Can you work these out from the model? Positions are in its coordinate system, mm. A direction names the side the tool comes from. Round coordinates to 2 decimals unless told otherwise and drop trailing zeros. Write each loop counter-clockwise with the first axis right and the second up, starting at its lowest first coordinate (ties: lowest second). Pieces come first, ordered by that corner, then holes.
Q1. We'd pull the mould along Y, two halves only. Please class faces 5 (the cylindrical face through (3.545, -3.18, 6.228)), 6 (the flat face through (0, 3.624, 3)), 7 (the flat face through (0, -3, 4.424)): +Y half, -Y half, draft (parallel to the pull), parting line (faces both ways), or undercut.
Q2. I'm going to push flat-ended pins straight in: pin 1 Ø0.8 at (x, y) = (0, -3) entering from +Z; pin 2 Ø1.1 at (x, z) = (-1, -0.5) entering from -Y; pin 3 Ø0.5 at (x, y) = (3, -3.5) entering from +Z; pin 4 Ø1.2 at (x, z) = (1, -1) entering from -Y. Where does each tip first touch, or does it pass through?
Q3. If we section it at A-A (z = 4.25): Please give me the cut outline in (x, y).
Q4. For faces 1 (the flat face through (0, -3.124, -1)), 2 (the cylindrical face through (-7.886, 0.069, -0.74)), 3 (the flat face through (0, 3.124, -1)), 4 (the cylindrical face through (6.926, -0.048, -0.291)), which set-ups out of +Z, -Z, +X, -X, +Y, -Y let a thin tool reach every point of the face, with its end or its side?
Q5. If we section it at B-B (y = 0): Please give me the cut outline in (x, z).
Q6. Please list where these lines run through material, in increasing order: line 1 along Y through (x, z) = (4.5, 3); line 2 along X through (y, z) = (0, 5.5); line 3 along Z through (x, y) = (-5.5, -1.25).
from build123d import *
from OCP.BRepAlgoAPI import BRepAlgoAPI_Cut
from OCP.TopTools import TopTools_ListOfShape

# Parameters (mm, degrees)
BOSS_EXTRUDE1_DEPTH      = 1.5
BOSS_EXTRUDE3_DEPTH      = 0.5
BOSS_EXTRUDE3_DRAFT      = -45
BOSS_EXTRUDE4_DEPTH      = 6.8
SHELL1_T                 = -0.96
SHELL1_THICKNESS_2_DEPTH = 0.46
CUT_EXTRUDE1_START       = -2.114122
CUT_EXTRUDE1_DEPTH       = 2.114122
SKETCH5_W                = 2.54
SKETCH5_H                = 7.2484
CUT_EXTRUDE2_DEPTH       = 0.762


with BuildPart() as part:
    # Sketch2 → Boss-Extrude1 (new body)
    with BuildSketch(Plane.XY):
        with BuildLine():
            Line((-4.7625, -3.1242), (4.7625, -3.1242))
            ThreePointArc((4.7625, -3.1242), (7.8867, 0), (4.7625, 3.1242))
            Line((4.7625, 3.1242), (-4.7625, 3.1242))
            ThreePointArc((-4.7625, 3.1242), (-7.8867, 0), (-4.7625, -3.1242))
        make_face()
    extrude(amount=-BOSS_EXTRUDE1_DEPTH)


with BuildPart() as boss_extrude3_tool:
    # Sketch2<3> → Boss-Extrude3 (with draft: the straight prism first)
    with BuildSketch(Plane.XY):
        with BuildLine():
            Line((-4.7625, -3.1242), (4.7625, -3.1242))
            ThreePointArc((4.7625, -3.1242), (7.8867, 0), (4.7625, 3.1242))
            Line((4.7625, 3.1242), (-4.7625, 3.1242))
            ThreePointArc((-4.7625, 3.1242), (-7.8867, 0), (-4.7625, -3.1242))
        make_face()
    extrude(amount=BOSS_EXTRUDE3_DEPTH)
    # Boss-Extrude3: the draft: its side faces are tilted about the plane it starts from
    boss_extrude3_sides = [boss_extrude3_tool.faces().sort_by_distance(p)[0] for p in [
        (0, -3.1242, 0.25),
        (7.8867, 0, 0.25),
        (0, 3.1242, 0.25),
        (-7.8867, 0, 0.25),
    ]]
    draft(boss_extrude3_sides, Plane.XY, BOSS_EXTRUDE3_DRAFT)


with BuildPart() as part_1:
    add(part.part)

    # Boss-Extrude3: add boss_extrude3_tool
    add(boss_extrude3_tool.part)

    # Sketch3 → Boss-Extrude4 (add)
    with BuildSketch(Plane.XY.offset(0.5)):
        with BuildLine():
            Line((-4.7625, -3.6242), (4.7625, -3.6242))
            ThreePointArc((4.7625, -3.6242), (8.3867, 0), (4.7625, 3.6242))
            Line((4.7625, 3.6242), (-4.7625, 3.6242))
            ThreePointArc((-4.7625, 3.6242), (-8.3867, 0), (-4.7625, -3.6242))
        make_face()
    extrude(amount=BOSS_EXTRUDE4_DEPTH)

    # Shell1
    shell1_openings = [part_1.faces().sort_by_distance(p)[0] for p in [
        (0, 0, 7.3),
    ]]
    offset(amount=SHELL1_T, openings=shell1_openings, kind=Kind.INTERSECTION)

    # Shell1 thickness 2 face (on inner face of the shell) → Shell1 thickness 2 (cut)
    with BuildSketch(Plane(origin=(0, 0, -0.54), x_dir=(-1, 0, 0), z_dir=(0, 0, -1))):
        with BuildLine():
            Line((-4.7625, 2.1642), (4.7625, 2.1642))
            ThreePointArc((4.7625, 2.1642), (6.9267, 0), (4.7625, -2.1642))
            Line((4.7625, -2.1642), (-4.7625, -2.1642))
            ThreePointArc((-4.7625, -2.1642), (-6.9267, 0), (-4.7625, 2.1642))
        make_face()
    extrude(amount=SHELL1_THICKNESS_2_DEPTH, mode=Mode.SUBTRACT)

    # Sketch4 → Cut-Extrude1 (cut)
    with BuildSketch(Plane.XY.offset(7.3).offset(CUT_EXTRUDE1_START)):
        with BuildLine():
            Line((1.3335, 4.572), (-1.3335, 4.572))
            ThreePointArc((-1.3335, 4.572), (-3.367596045, 3.367596045), (-4.572, 1.3335))
            Line((-4.572, 1.3335), (-4.572, -1.3335))
            ThreePointArc((-4.572, -1.3335), (-3.367596045, -3.367596045), (-1.3335, -4.572))
            Line((-1.3335, -4.572), (1.3335, -4.572))
            ThreePointArc((1.3335, -4.572), (3.367596045, -3.367596045), (4.572, -1.3335))
            Line((4.572, -1.3335), (4.572, 1.3335))
            ThreePointArc((4.572, 1.3335), (3.367596045, 3.367596045), (1.3335, 4.572))
        make_face()
    extrude(amount=CUT_EXTRUDE1_DEPTH, mode=Mode.SUBTRACT)


with BuildPart() as cut_extrude2_tool:
    # Sketch5 → Cut-Extrude2 (new body)
    with BuildSketch(Plane.XY.offset(5.185877531)):
        Rectangle(SKETCH5_W, SKETCH5_H)
    extrude(amount=-CUT_EXTRUDE2_DEPTH)


with BuildPart() as part_2:
    add(part_1.part)

    # Cut-Extrude2: cut by cut_extrude2_tool, with a tolerance
    cut_extrude2_stock = TopTools_ListOfShape()
    cut_extrude2_stock.Append(part_2.part.wrapped)
    cut_extrude2_tools = TopTools_ListOfShape()
    cut_extrude2_tools.Append(cut_extrude2_tool.part.wrapped)
    cut_extrude2_cut = BRepAlgoAPI_Cut()
    cut_extrude2_cut.SetArguments(cut_extrude2_stock)
    cut_extrude2_cut.SetTools(cut_extrude2_tools)
    cut_extrude2_cut.SetFuzzyValue(0.00001)
    cut_extrude2_cut.Build()
    add(Compound.cast(cut_extrude2_cut.Shape()).solids(), mode=Mode.REPLACE)


solid = part_2.part
A:
1. face 5: undercut
1. face 6: +Y half
1. face 7: draft
2. pin 1: stops at z = 4.42
2. pin 2: stops at y = -3.17
2. pin 3: stops at z = 7.3
2. pin 4: stops at y = -3.12
3. outline: (-4.76, -3.62) - (4.76, -3.62) arc R3.62 ccw to (4.76, 3.62) - (-4.76, 3.62) arc R3.62 ccw to start; hole (-4.76, -2.66) - (4.76, -2.66) arc R2.66 ccw to (4.76, 2.66) - (-4.76, 2.66) arc R2.66 ccw to start
4. face 1: -Z, +X, -X, -Y
4. face 2: -Z, -X
4. face 3: -Z, +X, -X, +Y
4. face 4: +Z
5. outline: (-8.39, 0.5) - (-7.89, 0) - (-7.89, -1.5) - (7.89, -1.5) - (7.89, 0) - (8.39, 0.5) - (8.39, 7.3) - (7.43, 7.3) - (7.43, 0.9) - (6.93, 0.4) - (6.93, -1) - (-6.93, -1) - (-6.93, 0.4) - (-7.43, 0.9) - (-7.43, 7.3) - (-8.39, 7.3) - close
6. line 1: y = -3.62 to -2.66, 2.66 to 3.62
6. line 2: x = -8.39 to -7.43, 7.43 to 8.39
6. line 3: z = -1.5 to -1
